Source: three-view drawing plus pictorial views. Frame: mm from the lowest corner of the part. A direction names the side the tool comes from. Give positions to 0.01 mm unless a question says otherwise; leave off trailing zeros. Loops run counter-clockwise (first coordinate to the right, second up) from the corner with the lowest first, then second, coordinate; pieces in that order, holes last. Notation, with made-up numbers: (6.5, -11.75) - (18.5, -11.75) arc R13 ccw to (18.5, 10.25) - close; hole circle Ø9 at (-19, 34.25). An arc over 180 degrees is marked (long way). One line per item, written item: value.
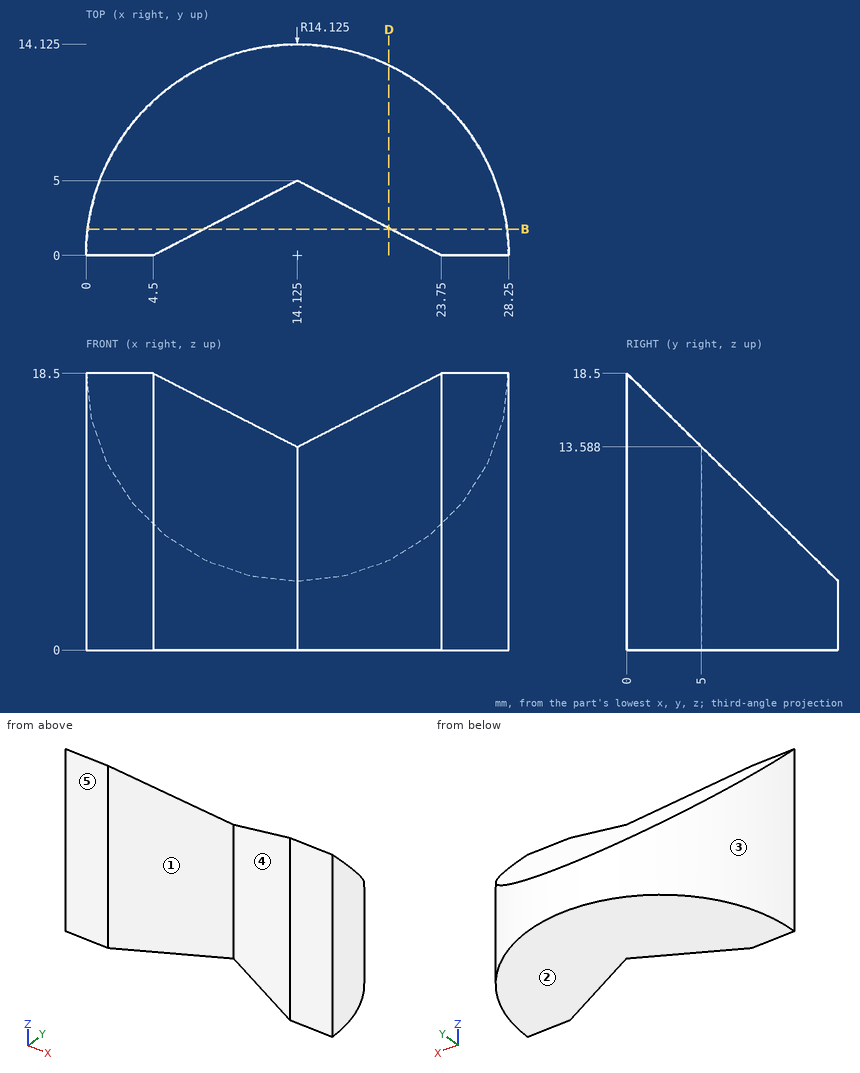
Item 1: Draft query along X for the marked faces 3, 4 and 5. Return one class per face: pulls with the +X half, pulls with the -X half, needs draft (parallel to the pull), parting line crosses it, or undercut.
Verdict:
face 3: parting line crosses it
face 4: undercut
face 5: needs draft
Item 2: Material intervals for L1, parallel to X at y = 4.5, z = 8 (1 decimal); L2, parallel to X at y = 4, z = 13; L3, parallel to Y at x = 23, z = 13, sorted ascending.
Verdict:
L1: x = 0.7 to 13.2, 15.1 to 27.5
L2: x = 0.58 to 12.2, 16.05 to 27.67
L3: y = 0.39 to 5.6
Item 3: Access query for the marked faces 1 and 2. Directions: +Z, -Z, +X, -X, +Y, -Y. A direction counts if a zero-diameter tool reaches every point of the face in a straight line with its end or side. Return the directions, or none.
Verdict:
face 1: +Z, -Z, -Y
face 2: -Z, +X, -X, +Y, -Y
Item 4: Section B-B, the plane y = 1.75. Output: boundary loops of the cut face in (x, z), and give its area (3 significant figures).
Verdict:
outline: (0.11, 0) - (7.87, 0) - (7.87, 16.78) - (0.11, 16.78) - close; (20.38, 0) - (28.14, 0) - (28.14, 16.78) - (20.38, 16.78) - close
area: 260 mm^2
Item 5: Section D-D, the plane x = 20.25. Output: boundary loops of the cut face in (y, z) (1 decimal).
Verdict:
outline: (1.8, 0) - (12.7, 0) - (12.7, 6) - (1.8, 16.7) - close
Item 6: Pin query (flat end, axial travel): P1, Ø4, axis at y = 8.5, z = 9, coming from the +X side (1 decimal); P2, Ø6, axis at y = 6, z = 15, coming from the +X side; P3, Ø1, axis at x = 20.5, z = 11, coming from the +Y side. Return the tip coordinate at first contact, or that it passes through.
Verdict:
P1: stops at x = 26.7
P2: stops at x = 27.93
P3: stops at y = 8.14
